```python
from build123d import *

# Parameters (mm, degrees)
SKETCH1_W           = 20
SKETCH1_H           = 96
BOSS_EXTRUDE2_DEPTH = 2
SKETCH3_R           = 1.75
SKETCH3_R_2         = 4.1
CUT_EXTRUDE1_DEPTH  = 50.071376586
CHAMFER1_SIZE       = 2


with BuildPart() as part:
    # Sketch1 → Boss-Extrude2 (new body)
    with BuildSketch(Plane(origin=(0, 0, 0), x_dir=(0, 0, -1), z_dir=(1, 0, 0))):
        Rectangle(SKETCH1_W, SKETCH1_H)
    extrude(amount=BOSS_EXTRUDE2_DEPTH)

    # Sketch3 → Cut-Extrude1 (cut, through all)
    with BuildSketch(Plane(origin=(2, 0, 0), x_dir=(0, 0, -1), z_dir=(1, 0, 0))):
        with Locations((0, 4.75)):
            Circle(SKETCH3_R)
        with Locations((0, -28)):
            Circle(SKETCH3_R_2)
        with BuildLine():
            ThreePointArc((3.099152102, 32.0725), (0, 43.75), (-3.099152102, 32.0725))
            ThreePointArc((-3.099152102, 32.0725), (0, 28.9), (3.099152102, 32.0725))
        make_face()
    extrude(amount=-CUT_EXTRUDE1_DEPTH, mode=Mode.SUBTRACT)

    # Chamfer1
    chamfer1_edges = [part.edges().sort_by_distance(p)[0] for p in [
        (1, -48, -10),
        (1, -48, 10),
        (1, 48, 10),
        (1, 48, -10),
    ]]
    chamfer(chamfer1_edges, length=CHAMFER1_SIZE)


solid = part.part
```
Could you check a few things on this model? Use its own coordinates, in mm. A direction names the side the tool comes from. Round coordinates to 2 decimals unless told otherwise and drop trailing zeros. Loops run counter-clockwise (first coordinate to the right, second up) from the corner with the lowest first, then second, coordinate; pieces in that order, holes last. Notation, with made-up numbers: (52, 41) -> (92, 41) arc R23 cw to (92, 62) -> close; hole circle Ø3 at (2.25, 4.5). An arc over 180 degrees is marked (long way). One line per question, with ' | ' between items.
(1) For pin 1 Ø1.5 at (y, z) = (-30, -6.5) entering from -X; pin 2 Ø7.5 at (y, z) = (-28, 0) entering from +X, each with a flat end and sliding along its axis, tell me the tip position at first contact or that it passes through.
Model answer:
pin 1: stops at x = 0 | pin 2: passes through
(2) Thinking about a two-plate mould opening in Y: for faces 3 (the face through (2, 1, 0)), 4 (the face through (1, 47, -9)), 5 (the face through (1, -32, 0.9)), 6 (the face through (1, -48, 0)), which applies, released by +Y, released by -Y, zero draft, split by the parting line, or undercut?
Model answer:
face 3: zero draft | face 4: released by +Y | face 5: undercut | face 6: released by -Y
(3) If we section it at B-B on z = 0: List the corners of the cut face in (x, y) for me.
Model answer:
outline: (0, -48) -> (2, -48) -> (2, -32.1) -> (0, -32.1) -> close; (0, -23.9) -> (2, -23.9) -> (2, 3) -> (0, 3) -> close; (0, 6.5) -> (2, 6.5) -> (2, 28.9) -> (0, 28.9) -> close; (0, 43.75) -> (2, 43.75) -> (2, 48) -> (0, 48) -> close
(4) If we section it at C-C on x = 1: List the corners of the cut face in (y, z) for me.
Model answer:
outline: (-48, -8) -> (-46, -10) -> (46, -10) -> (48, -8) -> (48, 8) -> (46, 10) -> (-46, 10) -> (-48, 8) -> close; hole circle Ø8.2 at (-28, 0); hole circle Ø3.5 at (4.75, 0); hole (32.07, -3.1) arc R6.25 ccw (long way) to (32.07, 3.1) arc R3.1 ccw (long way) to start
(5) For faces 1 (the face through (1, -1, 10)), 2 (the face through (1, 28.9, 0.1)), which set-ups out of +Z, -Z, +X, -X, +Y, -Y let a thin tool reach every point of the face, with its end or its side?
Model answer:
face 1: +Z, +X, -X, +Y, -Y | face 2: +X, -X
(6) If I drill on probe 1 along Y at (x, z) = (1.1, 0); probe 2 along Y at (x, z) = (0.25, 1); probe 3 along Y at (x, z) = (1.9, 2.75), over which ranges is the centre line in solid material (lowest first)?
Model answer:
probe 1: y = -48 to -32.1, -23.9 to 3, 6.5 to 28.9, 43.75 to 48 | probe 2: y = -48 to -31.98, -24.02 to 3.31, 6.19 to 29.07, 43.67 to 48 | probe 3: y = -48 to -31.04, -24.96 to 30.57, 43.11 to 48
(7) If we section it at A-A on y = 37.5: List the corners of the cut face in (x, z) for me, and give its area (3 significant figures).
Model answer:
outline: (0, -10) -> (2, -10) -> (2, -6.25) -> (0, -6.25) -> close; (0, 6.25) -> (2, 6.25) -> (2, 10) -> (0, 10) -> close | area: 15.0 mm^2
(8) If we section it at D-D on y = 4.75: List the corners of the cut face in (x, z) for me, and give its area (3 significant figures).
Model answer:
outline: (0, -10) -> (2, -10) -> (2, -1.75) -> (0, -1.75) -> close; (0, 1.75) -> (2, 1.75) -> (2, 10) -> (0, 10) -> close | area: 33.0 mm^2
